Build history of the part. All positions in model axes, mm. Round coordinates to 2 decimals unless told otherwise and drop trailing zeros. Loops run counter-clockwise (first coordinate to the right, second up) from the corner with the lowest first, then second, coordinate; pieces in that order, holes last. Notation, with made-up numbers: (75.5, 81) - (131.5, 81) arc R16 cw to (131.5, 93) - close; hole circle Ø2 at (50, 10.25). An arc over 180 degrees is marked (long way). Put each result on its own line as item: value. Start each with the question number.
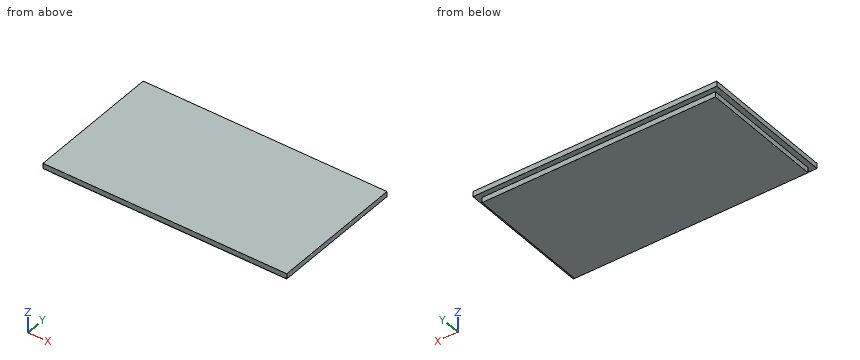
from build123d import *

# Parameters (mm, degrees)
SKETCH1_W           = 45
SKETCH1_H           = 24
BOSS_EXTRUDE1_DEPTH = 1
SKETCH2_W           = 47
SKETCH2_H           = 26
BOSS_EXTRUDE2_DEPTH = 1


with BuildPart() as part:
    # Sketch1 → Boss-Extrude1 (new body)
    with BuildSketch(Plane.XY.offset(40.959042005)):
        with Locations((18.613098235, 25.703029386)):
            Rectangle(SKETCH1_W, SKETCH1_H)
    extrude(amount=-BOSS_EXTRUDE1_DEPTH)

    # Sketch2 → Boss-Extrude2 (add)
    with BuildSketch(Plane.XY.offset(40.959042005)):
        with Locations((18.613098235, 25.703029386)):
            Rectangle(SKETCH2_W, SKETCH2_H)
    extrude(amount=BOSS_EXTRUDE2_DEPTH)


solid = part.part
Item 1: Drop flat-ended pins along their axis: pin 1 Ø0.8 at (x, z) = (27.5, 40.5) entering from +Y; pin 2 Ø0.5 at (x, z) = (20.5, 40.5) entering from -Y. Give the stop position or say it passes through.
Item 2: Slice it at C-C (z = 40.65). Give the cut face in (x, y).
Item 3: Drill centre lines: probe 1 along X at (y, z) = (34.75, 40.85); probe 2 along Y at (x, z) = (3, 40.65). Where is each one in solid material? Low to high. Write a range as [from, to].
Item 4: Slice it at B-B (y = 35.5). Give the cut face in (x, z), plus the area to 3 significant figures.
Item 5: Slice it at A-A (x = 23). Give the cut face in (y, z).
Computed values:
1. pin 1: stops at y = 37.7
1. pin 2: stops at y = 13.7
2. outline: (-3.89, 13.7) - (41.11, 13.7) - (41.11, 37.7) - (-3.89, 37.7) - close
3. probe 1: x = [-3.89, 41.11]
3. probe 2: y = [13.7, 37.7]
4. outline: (-4.89, 40.96) - (-3.89, 40.96) - (-3.89, 39.96) - (41.11, 39.96) - (41.11, 40.96) - (42.11, 40.96) - (42.11, 41.96) - (-4.89, 41.96) - close
4. area: 92.0 mm^2
5. outline: (12.7, 40.96) - (13.7, 40.96) - (13.7, 39.96) - (37.7, 39.96) - (37.7, 40.96) - (38.7, 40.96) - (38.7, 41.96) - (12.7, 41.96) - close
